Work out the finished part from the listing and answer in its coordinate system (mm). Face numbers are marked on the shaded views. A direction names the side the tool comes from. Give positions to 0.01 mm unless a question says otherwise; leave off trailing zeros. Loops run counter-clockwise (first coordinate to the right, second up) from the corner with the lowest first, then second, coordinate; pieces in that order, holes last. Notation, with made-up numbers: (64.5, -13) - (96.5, -13) arc R12 cw to (96.5, 5) - close; hole circle Ø3 at (36.5, -36). An arc over 180 degrees is marked (long way). One line per question, with ' | ' between items. Start each with the question number.
1. Each of these flat-tipped pins is pushed along its axis until it touches: pin 1 (4 mm diameter, centred on x = 1, z = -5.5, fed in from -Y); pin 2 (6 mm diameter, centred on y = 11, z = -3.5, fed in from +X); pin 3 (12 mm diameter, centred on y = 25, z = -17, fed in from -X); pin 4 (1 mm diameter, centred on x = -4.5, y = 18, fed in from -Z). Where does it stop, or does it pass through?
2. Section A-A (z = 0) is taken. Determine the outline of the cut face in (x, y), plus the area to 3 significant figures.
3. Find the intervals of material crossed by line 1 (X direction, y = 11.5, z = 0); line 2 (X direction, y = 10.5, z = 0); line 3 (X direction, y = 12.5, z = 2), in increasing order.
4. Which of the six approach directions +Z, -Z, +X, -X, +Y, -Y give full straight-line access (tool end or side, diameter ignored) to the marked faces 4 and 5?
5. Section B-B (x = 0) is taken. Determine the outline of the cut face in (y, z), plus the area to 3 significant figures.
6. Section D-D (y = 26.5) is taken. Determine the outline of the cut face in (x, z), plus the area to 3 significant figures.
7. Section C-C (y = 13.5) is taken. Determine the outline of the cut face in (x, z), plus the area to 3 significant figures.
8. For a pull along X with two mould halves and no side action, classify the marked faces 1, 2 and 3 as released by +X, released by -X, zero draft, split by the parting line, or undercut.
from build123d import *

# Parameters (mm, degrees)
SKETCH_2_R = 1.5
SKETCH_2_W = 10
SKETCH_2_H = 4


with BuildPart() as part:
    # 草图1 → 旋转1 (revolve)
    with BuildSketch(Plane.XY, mode=Mode.PRIVATE) as revolve_1_sk:
        Polygon((-12, 30), (-12, 15), (-30, 15), (-30, 0), (-6, 0), (-6, 30), align=None)
    revolve(revolve_1_sk.sketch.rotate(Axis((0, -28.507704651, 0), (0, 1, 0)), 270), axis=Axis((0, -28.507704651, 0), (0, 1, 0)))

    # 草图2 → 切除-旋转1 (revolve, cut)
    with BuildSketch(Plane.XY, mode=Mode.PRIVATE) as cut_revolve_1_sk:
        with Locations((-12, 24)):
            Circle(SKETCH_2_R)
        with Locations((-17, 13)):
            Rectangle(SKETCH_2_W, SKETCH_2_H)
        with Locations((-17, 2)):
            Rectangle(SKETCH_2_W, SKETCH_2_H)
    revolve(cut_revolve_1_sk.sketch.rotate(Axis((0, 0, 0), (0, 1, 0)), 270), axis=Axis((0, 0, 0), (0, 1, 0)), mode=Mode.SUBTRACT)


solid = part.part
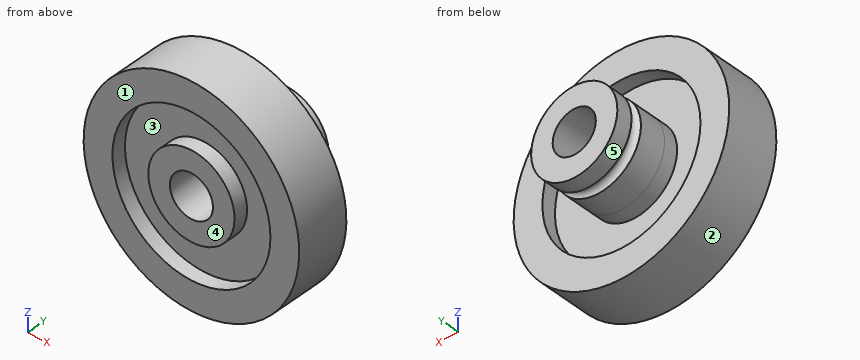
Conclusion:
1) pin 1: y = 0 | pin 2: x = 30 | pin 3: x = -4.75 | pin 4: z = -11.31
2) outline: (-30, 0) - (-22, 0) - (-22, 4) - (-12, 4) - (-12, 0) - (-6, 0) - (-6, 30) - (-12, 30) - (-12, 25.5) arc R1.5 cw to (-12, 22.5) - (-12, 11) - (-22, 11) - (-22, 15) - (-30, 15) - close; (6, 0) - (12, 0) - (12, 4) - (22, 4) - (22, 0) - (30, 0) - (30, 15) - (22, 15) - (22, 11) - (12, 11) - (12, 22.5) arc R1.5 cw to (12, 25.5) - (12, 30) - (6, 30) - close | area: 733 mm²
3) line 1: -30 to -22, -12 to -6, 6 to 12, 22 to 30 | line 2: -30 to -6, 6 to 30 | line 3: -29.93 to -21.91, -11.83 to -5.66, 5.66 to 11.83, 21.91 to 29.93
4) face 4: +Z, -Z, +X, -X, -Y | face 5: +Y
5) outline: (0, -30) - (15, -30) - (15, -22) - (11, -22) - (11, -12) - (22.5, -12) arc R1.5 cw to (25.5, -12) - (30, -12) - (30, -6) - (0, -6) - (0, -12) - (4, -12) - (4, -22) - (0, -22) - close; (0, 6) - (30, 6) - (30, 12) - (25.5, 12) arc R1.5 cw to (22.5, 12) - (11, 12) - (11, 22) - (15, 22) - (15, 30) - (0, 30) - (0, 22) - (4, 22) - (4, 12) - (0, 12) - close | area: 733 mm²
6) outline: circle Ø24 at (0, 0); hole circle Ø12 at (0, 0) | area: 339 mm²
7) outline: circle Ø60 at (0, 0); circle Ø24 at (0, 0); hole circle Ø44 at (0, 0); hole circle Ø12 at (0, 0) | area: 1,650 mm²
8) face 1: zero draft | face 2: split by the parting line | face 3: undercut
